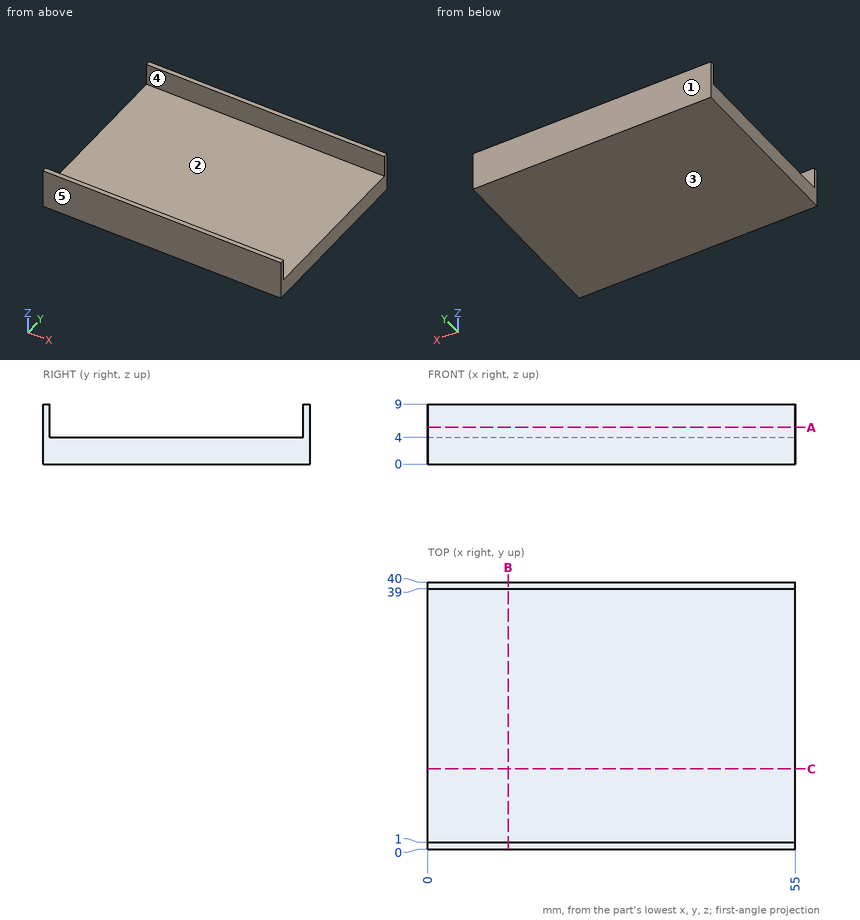
Source: three-view drawing plus pictorial views. Frame: mm from the lowest corner of the part. A direction names the side the tool comes from. Round coordinates to 2 decimals unless told otherwise and drop trailing zeros. Loops run counter-clockwise (first coordinate to the right, second up) from the corner with the lowest first, then second, coordinate; pieces in that order, holes last.
Q1. Section A-A, the plane z = 5.5. Return loops of the section in (x, y), plus the area to 3 significant figures.
Q2. Mould query, pull axis Y, two halves, no side actions, for the marked faces 3, 4 and 5. Classes: pulls with the +Y half, pulls with the -Y half, needs draft (parallel to the pull), parting line crosses it, or undercut.
Q3. Section B-B, the plane x = 12. Return loops of the section in (y, z).
Q4. Ray query, line 1 (Y direction, x = 33.5, z = 6.75); line 2 (Z direction, x = 40.5, y = 31). Return the intervals inside material, ascending.
Q5. First-contact query: P1, Ø4, axis at x = 31, y = 33, coming from the +Z side. Flat tip, straight axial feed; report the tip coordinate or a pass-through.
Q6. Access query for the marked faces 1 and 2. Directions: +Z, -Z, +X, -X, +Y, -Y. A direction counts if a zero-diameter tool reaches every point of the face in a straight line with its end or side. Return the directions, or none.
Q7. Section C-C, the plane y = 12. Return loops of the section in (x, z).
Solutions:
1. outline: (0, 0) - (55, 0) - (55, 1) - (0, 1) - close; (0, 39) - (55, 39) - (55, 40) - (0, 40) - close
1. area: 110 mm2
2. face 3: needs draft
2. face 4: undercut
2. face 5: pulls with the -Y half
3. outline: (0, 0) - (40, 0) - (40, 9) - (39, 9) - (39, 4) - (1, 4) - (1, 9) - (0, 9) - close
4. line 1: y = 0 to 1, 39 to 40
4. line 2: z = 0 to 4
5. P1: stops at z = 4
6. face 1: +Z, -Z, +X, -X, +Y
6. face 2: +Z, +X, -X
7. outline: (0, 0) - (55, 0) - (55, 4) - (0, 4) - close
